The model under review builds one solid part; all positions refer to its coordinate system, in mm. Face numbers are marked on the shaded views. A direction names the side the tool comes from. Give positions to 0.01 mm unless a question says otherwise; leave off trailing zeros. Loops run counter-clockwise (first coordinate to the right, second up) from the corner with the lowest first, then second, coordinate; pieces in that order, holes last. Notation, with made-up numbers: (39, 65) - (46, 65) arc R18 ccw to (46, 86) - close; hole circle Ø1 at (-6, -7.5). An arc over 180 degrees is marked (long way). Answer as a JSON object with one key per item and string values.
from build123d import *

# Parameters (mm, degrees)
SKETCH_1_W          = 125
SKETCH_1_H          = 49
EXTRUDE_1_DEPTH     = 25
SKETCH_2_OUTSIDE_W  = 154.314
SKETCH_2_OUTSIDE_H  = 54.314
CUT_EXTRUDE_1_DEPTH = 84.260134518
SKETCH_3_R          = 2.1
CUT_EXTRUDE_2_DEPTH = 25


with BuildPart() as part:
    # 草图1 → 凸台-拉伸1 (new body)
    with BuildSketch(Plane(origin=(0, 0, 0), x_dir=(1, 0, 0), z_dir=(0, 1, 0))):
        Rectangle(SKETCH_1_W, SKETCH_1_H)
    extrude(amount=EXTRUDE_1_DEPTH)

    # 草图2 outside → 切除-拉伸1 (cut, through all)
    with BuildSketch(Plane.XY.offset(24.5)):
        with Locations((0, 12.5)):
            Rectangle(SKETCH_2_OUTSIDE_W, SKETCH_2_OUTSIDE_H)
        Polygon((-62.5, 1.5), (-49.5, 1.5), (-49.5, 5.5), (-40, 25), (40, 25), (49.5, 5.5), (49.5, 1.5), (62.5, 1.5), (62.5, 0), (-62.5, 0), align=None, mode=Mode.SUBTRACT)
    extrude(amount=-CUT_EXTRUDE_1_DEPTH, mode=Mode.SUBTRACT)

    # 草图3 → 切除-拉伸2 (cut)
    with BuildSketch(Plane.XZ):
        with Locations(Location((-57.5, 0, 0), (0, 0, 270))):
            Circle(SKETCH_3_R)
        with Locations(Location((57.5, 0, 0), (0, 0, 180))):
            Circle(SKETCH_3_R)
        with BuildLine():
            Line((-62.5, 16.6), (-57.5, 16.6))
            ThreePointArc((-57.5, 16.6), (-55.4, 14.5), (-57.5, 12.4))
            Line((-57.5, 12.4), (-62.5, 12.4))
            Line((-62.5, 12.4), (-62.5, 16.6))
        make_face()
        with BuildLine():
            Line((62.5, 16.6), (62.5, 12.4))
            Line((62.5, 12.4), (57.5, 12.4))
            ThreePointArc((57.5, 12.4), (55.4, 14.5), (57.5, 16.6))
            Line((57.5, 16.6), (62.5, 16.6))
        make_face()
        with BuildLine():
            Line((62.5, -16.6), (57.5, -16.6))
            ThreePointArc((57.5, -16.6), (55.4, -14.5), (57.5, -12.4))
            Line((57.5, -12.4), (62.5, -12.4))
            Line((62.5, -12.4), (62.5, -16.6))
        make_face()
        with BuildLine():
            Line((-62.5, -16.6), (-62.5, -12.4))
            Line((-62.5, -12.4), (-57.5, -12.4))
            ThreePointArc((-57.5, -12.4), (-55.4, -14.5), (-57.5, -16.6))
            Line((-57.5, -16.6), (-62.5, -16.6))
        make_face()
    extrude(amount=-CUT_EXTRUDE_2_DEPTH, mode=Mode.SUBTRACT)


solid = part.part
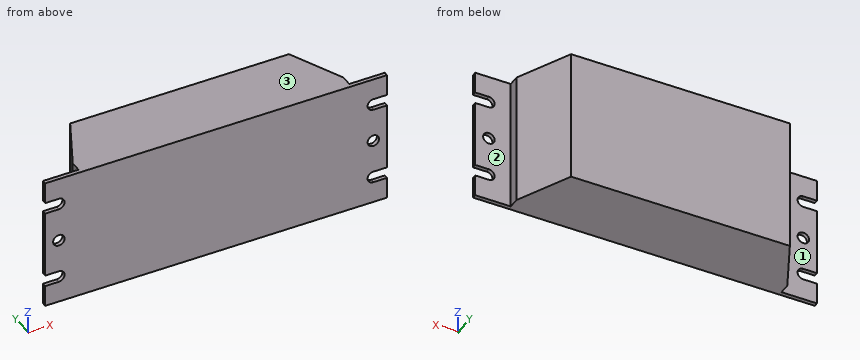
Q1. Consider section C-C, the plane x = -53. State the section outline as (y, z) points.
Results:
{"outline": "(0, -24.5) - (1.5, -24.5) - (1.5, 24.5) - (0, 24.5) - close"}
Q2. Consider section D-D, the plane z = -6. State the section outline as (x, y) points, plus the area to 3 significant figures.
Results:
{"outline": "(-62.5, 0) - (62.5, 0) - (62.5, 1.5) - (49.5, 1.5) - (49.5, 5.5) - (40, 25) - (-40, 25) - (-49.5, 5.5) - (-49.5, 1.5) - (-62.5, 1.5) - close", "area": "2,330 mm^2"}
Q3. Consider section B-B, the plane z = 14.5. State the section outline as (x, y) points.
Results:
{"outline": "(-55.4, 0) - (55.4, 0) - (55.4, 1.5) - (49.5, 1.5) - (49.5, 5.5) - (40, 25) - (-40, 25) - (-49.5, 5.5) - (-49.5, 1.5) - (-55.4, 1.5) - close"}
Q4. To check wall thickness, follow probe 1 along Z at (x, y) = (57.5, 0.4); probe 2 along Y at (x, z) = (-52.5, 16.5); probe 3 along Y at (x, z) = (48, 9). State the ranges of each line that lie inside material, in increasing order. Write a range as [from, to].
Results:
{"probe 1": "z = [-24.5, -16.6], [-12.4, -2.1], [2.1, 12.4], [16.6, 24.5]", "probe 2": "y = [0, 1.5]", "probe 3": "y = [0, 8.58]"}
Q5. Consider section A-A, the plane z = 0. State the section outline as (x, y) points.
Results:
{"outline": "(-62.5, 0) - (-59.6, 0) - (-59.6, 1.5) - (-62.5, 1.5) - close; (-55.4, 0) - (55.4, 0) - (55.4, 1.5) - (49.5, 1.5) - (49.5, 5.5) - (40, 25) - (-40, 25) - (-49.5, 5.5) - (-49.5, 1.5) - (-55.4, 1.5) - close; (59.6, 0) - (62.5, 0) - (62.5, 1.5) - (59.6, 1.5) - close"}
Q6. For the marked faces 1, 2 and 3, list the 3-axis set-ups (+Z, -Z, +X, -X, +Y, -Y) from which the entire face can be reached by the end or side of a thin tool; tool diameter is ignored.
Results:
{"face 1": "+Z, -Z, -X, +Y", "face 2": "+Z, -Z, +X, +Y", "face 3": "+Z, +X, -X, +Y, -Y"}
Q7. Clearance check with flat-ended pins moving along their axes: pin 1 Ø2 at (y, z) = (3.5, -1) entering from +X; pin 2 Ø14.5 at (x, z) = (-58.5, 7.5) entering from +Y; pin 3 Ø4 at (y, z) = (10, -3) entering from +X. State where each tip first meets the part, or that it passes through.
Results:
{"pin 1": "stops at x = 49.5", "pin 2": "stops at y = 1.5", "pin 3": "stops at x = 48.28"}
